Geometry: final body of the model. Coordinates: model frame, mm. A direction names the side the tool comes from. Give positions to 0.01 mm unless a question says otherwise; leave off trailing zeros. Write each loop counter-clockwise with the first axis right and the second up, starting at its lowest first coordinate (ties: lowest second). Pieces come first, ordered by that corner, then holes. Notation, with made-up numbers: (-9.75, -21) -> (10.25, -21) arc R25 cw to (10.25, 15) -> close; hole circle Ø1 at (-39, 58). An arc over 180 degrees is marked (long way). Use CSV: the item, a comma, the result in double quotes. Start each with the question number.
1) Contact query for flat-ended pins moving along their axis: P1, Ø6, axis at x = -2, z = 5, coming from the +Y side; P2, Ø8, axis at x = 0, z = 0, coming from the -Y side; P3, Ø6, axis at y = 9, z = -9.5, coming from the -X side. Output: stop coordinate, or through.
2) Section D-D (z = -6.25). Output: boundary loops of the cut face in (x, y).
3) Section B-B (z = -1.75). Output: boundary loops of the cut face in (x, y), plus the area to 3 significant figures.
4) Section C-C (x = 5.5). Output: boundary loops of the cut face in (y, z).
5) Material intervals for line 1 (Z direction, x = 8.5, y = 18); line 2 (X direction, y = 3.65, z = 0); line 3 (Y direction, x = -7.25, z = 7), sorted ascending. Write a range as [from, to].
6) Set-up query: faces 4 (the face through (-0.52, 23.64, 0.14)), 5 (the face through (-4.88, 2.46, -1.08)), 6 (the face through (-7.15, 31.99, 10.99)). Return all of +Z, -Z, +X, -X, +Y, -Y with unobstructed straight access to the full face (end or side cutting, diameter ignored); none if empty.
7) Draft query along Y for faces 1 (the face through (-2, 5, -5)), 2 (the face through (-5, 0, -3)), 3 (the face through (7.15, 31.99, -11.01)). Return one class per face: pulls with the +Y half, pulls with the -Y half, needs draft (parallel to the pull), parting line crosses it, or undercut.
8) Section A-A (y = 14). Output: boundary loops of the cut face in (x, z).
```python
from build123d import *

# Parameters (mm, degrees)
SKETCH1_W                = 20
SKETCH1_H                = 20
SKETCH1_R                = 5
BOSS_EXTRUDE1_DEPTH      = 5
BOSS_EXTRUDE2_DEPTH      = 30
BOSS_EXTRUDE2_DEPTH_BACK = 5
SKETCH2_W                = 20
SKETCH2_H                = 2
FILLET1_R                = 10
SKETCH4_R                = 4
BOSS_EXTRUDE4_DEPTH      = 20


with BuildPart() as part:
    # Sketch1 → Boss-Extrude1 (new body)
    with BuildSketch(Plane(origin=(0, 0, 0), x_dir=(1, 0, 0), z_dir=(0, 1, 0))):
        Rectangle(SKETCH1_W, SKETCH1_H)
        with Locations(Location((0, 0, 0), (0, 0, 270))):
            Circle(SKETCH1_R, mode=Mode.SUBTRACT)
    extrude(amount=BOSS_EXTRUDE1_DEPTH)

    # Sketch2 → Boss-Extrude2 (add, two sides: drawn at the far end of the back side and taken through both)
    with BuildSketch(Plane(origin=(0, 5, 0), x_dir=(1, 0, 0), z_dir=(0, 1, 0)).offset(-BOSS_EXTRUDE2_DEPTH_BACK)):
        with Locations((0, -11)):
            Rectangle(SKETCH2_W, SKETCH2_H)
        with Locations((0, 11)):
            Rectangle(SKETCH2_W, SKETCH2_H)
    extrude(amount=BOSS_EXTRUDE2_DEPTH + BOSS_EXTRUDE2_DEPTH_BACK)

    # Fillet1
    fillet1_edges = [part.edges().sort_by_distance(p)[0] for p in [
        (10, 35, -11),
        (10, 35, 11),
        (-10, 35, 11),
        (-10, 35, -11),
    ]]
    fillet(fillet1_edges, radius=FILLET1_R - 0.0001)  # a hair under: the kernel refuses the full size

    # Sketch4 → Boss-Extrude4 (add)
    with BuildSketch(Plane(origin=(0, 0, 10), x_dir=(-1, 0, 0), z_dir=(0, 0, -1))):
        with Locations(Location((0, 27.604071929, 0), (0, 0, 180))):
            Circle(SKETCH4_R)
    extrude(amount=BOSS_EXTRUDE4_DEPTH)


solid = part.part
```
Answers follow:
1,P1,"stops at y = 31.6"
1,P2,"stops at y = 23.6"
1,P3,"stops at x = -10"
2,outline,"(-10, 0) -> (10, 0) -> (10, 5) -> (-10, 5) -> close; circle Ø8 at (0, 27.6)"
3,outline,"(-10, 0) -> (-4.68, 0) -> (-4.68, 5) -> (-10, 5) -> close; circle Ø8 at (0, 27.6); (4.68, 0) -> (10, 0) -> (10, 5) -> (4.68, 5) -> close"
3,area,"103 mm^2"
4,outline,"(0, -12) -> (33.35, -12) -> (33.35, -10) -> (5, -10) -> (5, 10) -> (33.35, 10) -> (33.35, 12) -> (0, 12) -> close"
5,line 1,"z = [-12, -10], [10, 12]"
5,line 2,"x = [-10, -5], [5, 10]"
5,line 3,"y = [0, 5]"
6,face 4,"none"
6,face 5,"-Y"
6,face 6,"+Z, -Z, -X, +Y"
7,face 1,"undercut"
7,face 2,"pulls with the -Y half"
7,face 3,"pulls with the +Y half"
8,outline,"(-10, -12) -> (10, -12) -> (10, -10) -> (-10, -10) -> close; (-10, 10) -> (10, 10) -> (10, 12) -> (-10, 12) -> close"
